```python
from build123d import *

# Parameters (mm, degrees)
F0_R          = 1.25
F1_DEPTH      = 4.5
F3_R          = 2
F4_DEPTH      = 3.9
F4_DEPTH_BACK = 40.9


with BuildPart() as f1:
    # F0 (on Top) → F1 (new body)
    with BuildSketch(Plane.XY):
        Polygon((19, 31.5), (-19, 31.5), (-18.5, -31.5), (18.5, -31.5), align=None)
        with Locations((-9.525, -27.94)):
            Circle(F0_R, mode=Mode.SUBTRACT)
        with Locations((9.525, -27.94)):
            Circle(F0_R, mode=Mode.SUBTRACT)
        with Locations((-9.525, 27.94)):
            Circle(F0_R, mode=Mode.SUBTRACT)
        with Locations((9.525, 27.94)):
            Circle(F0_R, mode=Mode.SUBTRACT)
    extrude(amount=F1_DEPTH)

    # F3 (on offset) → F4 (join, two sides)
    with BuildSketch(Plane(origin=(18.7488190464, -0.1488001512, 0), x_dir=(0.007936258, 0.9999685074, 0), z_dir=(0.9999685074, -0.007936258, 0))) as f4_sk:
        with Locations((13.6478127895, 2.25)):
            Circle(F3_R)
        with Locations((-13.3521872105, 2.25)):
            Circle(F3_R)
    extrude(amount=F4_DEPTH)
    extrude(f4_sk.sketch, amount=-F4_DEPTH_BACK)


solid = f1.part
```
Input: part model. Units: mm. Frame: model coordinates. Round coordinates to 2 decimals unless told otherwise and drop trailing zeros. Loops run counter-clockwise (first coordinate to the right, second up) from the corner with the lowest first, then second, coordinate; pieces in that order, holes last. Notation, with made-up numbers: (22, 57) -> (52, 57) arc R12 ccw to (52, 78) -> close; hole circle Ø7 at (0.25, 26). An arc over 180 degrees is marked (long way). One line per item, written item: value.
(1) Section A-A (z = 2.95). Return the cut outline in (x, y) (3 decimals), plus the area to 3 significant figures.
Geometry check:
outline: (-22.271, -15.049) -> (-18.63, -15.078) -> (-18.5, -31.5) -> (18.5, -31.5) -> (18.628, -15.374) -> (22.528, -15.405) -> (22.558, -11.658) -> (18.658, -11.627) -> (18.842, 11.625) -> (22.742, 11.594) -> (22.772, 15.341) -> (18.872, 15.372) -> (19, 31.5) -> (-19, 31.5) -> (-18.874, 15.672) -> (-22.027, 15.697) -> (-22.056, 11.95) -> (-18.845, 11.924) -> (-18.66, -11.331) -> (-22.241, -11.303) -> close; hole circle Ø2.5 at (-9.525, -27.94); hole circle Ø2.5 at (-9.525, 27.94); hole circle Ø2.5 at (9.525, -27.94); hole circle Ø2.5 at (9.525, 27.94)
area: 2,400 mm2
(2) Material intervals for line 1 (X direction, y = 28, z = 3.3); line 2 (X direction, y = -12.5, z = 2.2); line 3 (Y direction, x = 20, z = 2.1), sorted ascending. Write a range as [from, to].
Geometry check:
line 1: [-18.97, -10.77], [-8.28, 8.28], [10.77, 18.97]
line 2: [-22.25, 22.55]
line 3: [-15.51, -11.52], [11.5, 15.48]
(3) Section D-D (y = -6). Return the cut outline in (x, z), plus the area to 3 significant figures.
Geometry check:
outline: (-18.7, 0) -> (18.7, 0) -> (18.7, 4.5) -> (-18.7, 4.5) -> close
area: 168 mm2
(4) Mould query, pull axis X, two halves, no side actions, for faces 1 (the face through (0, -31.5, 2)), 2 (the face through (-9.8, -29.16, 2.22)). Classes: pulls with the +X half, pulls with the -X half, needs draft (parallel to the pull), parting line crosses it, or undercut.
Geometry check:
face 1: needs draft
face 2: undercut
(5) Pin query (flat end, axial travel): pin 1 (2 mm diameter, centred on x = -9.525, y = -27.94, fed in from -Z); pin 2 (1 mm diameter, centred on y = 18.5, z = 1.5, fed in from -X). Return the tip coordinate at first contact, or that it passes through.
Geometry check:
pin 1: through
pin 2: x = -18.9
(6) Section B-B (y = -27.94). Return the cut outline in (x, z) (3 decimals).
Geometry check:
outline: (-18.528, 0) -> (-10.775, 0) -> (-10.775, 4.5) -> (-18.528, 4.5) -> close; (-8.275, 0) -> (8.275, 0) -> (8.275, 4.5) -> (-8.275, 4.5) -> close; (10.775, 0) -> (18.528, 0) -> (18.528, 4.5) -> (10.775, 4.5) -> close
(7) Section C-C (y = 27.94). Return the cut outline in (x, z) (3 decimals), plus the area to 3 significant figures.
Geometry check:
outline: (-18.972, 0) -> (-10.775, 0) -> (-10.775, 4.5) -> (-18.972, 4.5) -> close; (-8.275, 0) -> (8.275, 0) -> (8.275, 4.5) -> (-8.275, 4.5) -> close; (10.775, 0) -> (18.972, 0) -> (18.972, 4.5) -> (10.775, 4.5) -> close
area: 148 mm2
